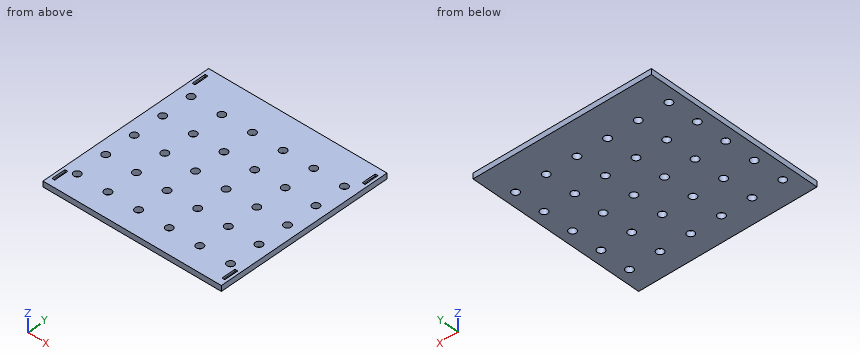
from build123d import *

# Parameters (mm, degrees)
CROQUIS1_W              = 640
CROQUIS1_H              = 640
SALIENTE_EXTRUIR1_DEPTH = 20
CROQUIS2_W              = 10.1
CROQUIS2_H              = 50.1
CORTAR_EXTRUIR1_DEPTH   = 8
CROQUIS3_R              = 13
CORTAR_EXTRUIR2_DEPTH   = 48


with BuildPart() as part:
    # Croquis1 → Saliente-Extruir1 (new body)
    with BuildSketch(Plane.XY):
        Rectangle(CROQUIS1_W, CROQUIS1_H)
    extrude(amount=SALIENTE_EXTRUIR1_DEPTH)

    # Croquis2 → Cortar-Extruir1 (cut)
    with BuildSketch(Plane.XY.offset(20)):
        with Locations((-305.05, 270.931721093)):
            Rectangle(CROQUIS2_W, CROQUIS2_H)
        with Locations((305.05, 270.931721093)):
            Rectangle(CROQUIS2_W, CROQUIS2_H)
    cortar_extruir1 = extrude(amount=-CORTAR_EXTRUIR1_DEPTH, mode=Mode.SUBTRACT)

    # Simetría1: Cortar-Extruir1 across plane
    add(cortar_extruir1.mirror(Plane.ZX), mode=Mode.SUBTRACT)

    # Croquis3 → Cortar-Extruir2 (cut)
    with BuildSketch(Plane.XY.offset(20)):
        with Locations((-274.388478244, 203.250724625)):
            Circle(CROQUIS3_R)
        with Locations((-164.388478244, 203.250724625)):
            Circle(CROQUIS3_R)
        with Locations((-54.388478244, 203.250724625)):
            Circle(CROQUIS3_R)
        with Locations((55.611521756, 203.250724625)):
            Circle(CROQUIS3_R)
        with Locations((165.611521756, 203.250724625)):
            Circle(CROQUIS3_R)
        with Locations((275.611521756, 203.250724625)):
            Circle(CROQUIS3_R)
        with Locations((-164.388478244, 93.250724625)):
            Circle(CROQUIS3_R)
        with Locations((-54.388478244, 93.250724625)):
            Circle(CROQUIS3_R)
        with Locations((55.611521756, 93.250724625)):
            Circle(CROQUIS3_R)
        with Locations((165.611521756, 93.250724625)):
            Circle(CROQUIS3_R)
        with Locations((275.611521756, 93.250724625)):
            Circle(CROQUIS3_R)
        with Locations((-164.388478244, -16.749275375)):
            Circle(CROQUIS3_R)
        with Locations((-54.388478244, -16.749275375)):
            Circle(CROQUIS3_R)
        with Locations((55.611521756, -16.749275375)):
            Circle(CROQUIS3_R)
        with Locations((165.611521756, -16.749275375)):
            Circle(CROQUIS3_R)
        with Locations((275.611521756, -16.749275375)):
            Circle(CROQUIS3_R)
        with Locations((-164.388478244, -126.749275375)):
            Circle(CROQUIS3_R)
        with Locations((-54.388478244, -126.749275375)):
            Circle(CROQUIS3_R)
        with Locations((55.611521756, -126.749275375)):
            Circle(CROQUIS3_R)
        with Locations((165.611521756, -126.749275375)):
            Circle(CROQUIS3_R)
        with Locations((275.611521756, -126.749275375)):
            Circle(CROQUIS3_R)
        with Locations((-164.388478244, -236.749275375)):
            Circle(CROQUIS3_R)
        with Locations((-54.388478244, -236.749275375)):
            Circle(CROQUIS3_R)
        with Locations((55.611521756, -236.749275375)):
            Circle(CROQUIS3_R)
        with Locations((165.611521756, -236.749275375)):
            Circle(CROQUIS3_R)
        with Locations((275.611521756, -236.749275375)):
            Circle(CROQUIS3_R)
        with Locations((-274.388478244, 93.250724625)):
            Circle(CROQUIS3_R)
        with Locations((-274.388478244, -16.749275375)):
            Circle(CROQUIS3_R)
        with Locations((-274.388478244, -126.749275375)):
            Circle(CROQUIS3_R)
        with Locations((-274.388478244, -236.749275375)):
            Circle(CROQUIS3_R)
    extrude(amount=-CORTAR_EXTRUIR2_DEPTH, mode=Mode.SUBTRACT)


solid = part.part
The model under review builds one solid part; all positions refer to its coordinate system, in mm. Round coordinates to 2 decimals unless told otherwise and drop trailing zeros. Order: outer loops, then holes, each group sorted by start corner. A loop starts at its lowest first (then second) coordinate and runs counter-clockwise, first axis right, second up. Notation, with made-up numbers: (42.25, -38) - (92.25, -38) arc R22 cw to (92.25, -16) - close; hole circle Ø2 at (-14, 89). An arc over 180 degrees is marked (long way). Use one line per item in the form item = value.
Q1. To check wall thickness, follow line 1 (X direction, y = 247, z = 14.75); line 2 (Y direction, x = 160.5, z = 4.75); line 3 (Y direction, x = 60, z = 13.25). State the ranges of each line that lie inside material, in increasing order.
Response values:
line_1 = -320 to -310.1, -300 to 300, 310.1 to 320
line_2 = -320 to -248.7, -224.8 to -138.7, -114.8 to -28.7, -4.8 to 81.3, 105.2 to 191.3, 215.2 to 320
line_3 = -320 to -248.99, -224.51 to -138.99, -114.51 to -28.99, -4.51 to 81.01, 105.49 to 191.01, 215.49 to 320
Q2. Add section B-B on z = 8.5. Give the number of separate pieces and of enclosed holes in the cut face, then the cut area to 3 significant figures.
Response values:
separate_pieces = 1
enclosed_holes = 30
area = 394,000 mm^2
Q3. Add section A-A on x = 58.5. Give the boundary of the cut face in (y, z), then the cut area to 3 significant figures.
Response values:
outline = (-320, 0) - (-249.42, 0) - (-249.42, 20) - (-320, 20) - close; (-224.07, 0) - (-139.42, 0) - (-139.42, 20) - (-224.07, 20) - close; (-114.07, 0) - (-29.42, 0) - (-29.42, 20) - (-114.07, 20) - close; (-4.07, 0) - (80.58, 0) - (80.58, 20) - (-4.07, 20) - close; (105.93, 0) - (190.58, 0) - (190.58, 20) - (105.93, 20) - close; (215.93, 0) - (320, 0) - (320, 20) - (215.93, 20) - close
area = 10,300 mm^2
Q4. Clearance check with a flat-ended pin moving along its axis: P1, Ø5, axis at x = 307, y = -266.5, coming from the +Z side. State where the tip first meets the part, or that it passes through.
Response values:
P1 = 12
